Job drawing, mm, ordinate dimensions from the low corner. One solid piece. Give positions to 0.01 mm unless a question says otherwise; leave off trailing zeros. Loops run counter-clockwise (first coordinate to the right, second up) from the corner with the lowest first, then second, coordinate; pieces in that order, holes last. Notation, with made-up numbers: M 35.5,58 L 65.5,58 A31 ccw 65.5,94 Z; hole C 47.5,-2.5 d9. An arc over 180 degrees is marked long. Put each result on its own line as item: value.
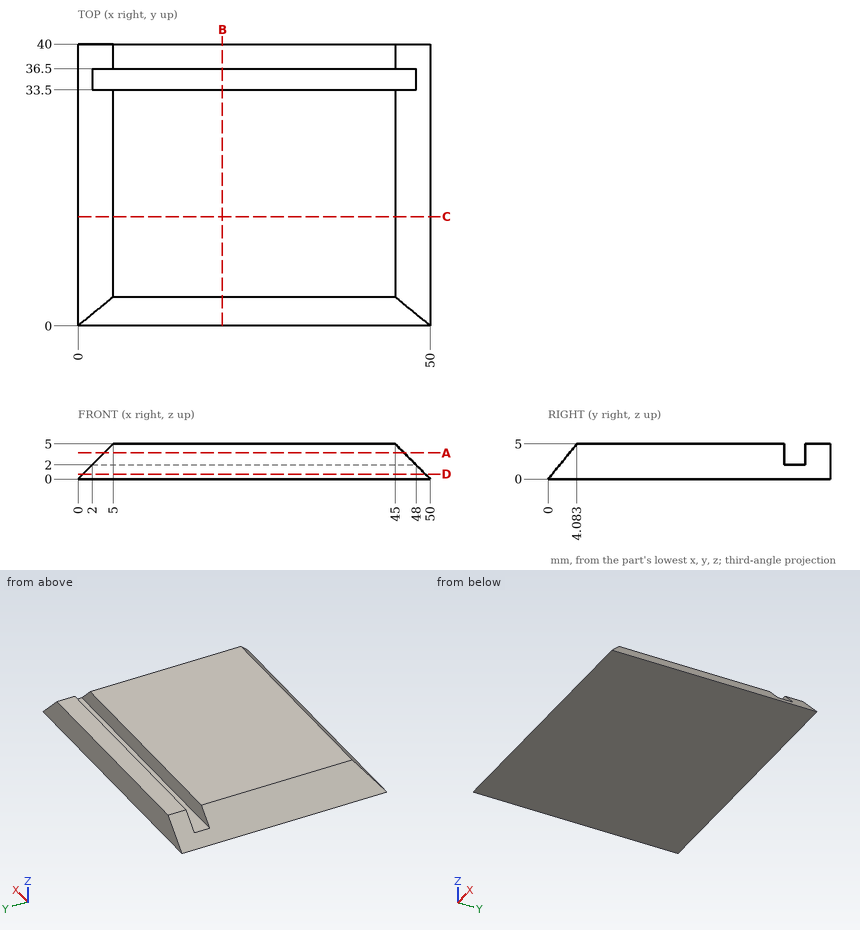
Q1. Slice it at A-A (z = 3.7). List the corners of the cut face in (x, y).
Here are the results:
outline: M 3.7,3.02 L 46.3,3.02 L 46.3,33.5 L 3.7,33.5 Z; M 3.7,36.5 L 46.3,36.5 L 46.3,40 L 3.7,40 Z
Q2. Slice it at D-D (z = 0.7). List the corners of the cut face in (x, y), and give its area (3 significant figures).
Here are the results:
outline: M 0.7,0.57 L 49.3,0.57 L 49.3,40 L 0.7,40 Z
area: 1,920 mm²
Q3. Probe line 1 (Z direction, x = 45, y = 34); line 2 (Y direction, x = 31.5, z = 2.25); line 3 (Y direction, x = 11.5, z = 3.9) (1 decimal). List the from-to ranges inside material, lowest first. Write a range as from..to.
Here are the results:
line 1: 0..2
line 2: 1.84..33.5, 36.5..40
line 3: 3.2..33.5, 36.5..40
Q4. Slice it at C-C (y = 15.5). List the corners of the cut face in (x, z).
Here are the results:
outline: M 0,0 L 50,0 L 45,5 L 5,5 Z
Q5. Slice it at B-B (x = 20.5). List the corners of the cut face in (y, z).
Here are the results:
outline: M 0,0 L 40,0 L 40,5 L 36.5,5 L 36.5,2 L 33.5,2 L 33.5,5 L 4.08,5 Z
Q6. Drop flat-ended pins along their axis: pin 1 Ø1.5 at (x, z) = (24.5, 2.5) entering from -Y; pin 2 Ø2 at (x, z) = (13.5, 2) entering from -Y; pin 3 Ø0.9 at (x, y) = (19, 35) entering from +Z. Give the stop position or say it passes through.
Here are the results:
pin 1: y = 1.43
pin 2: y = 0.82
pin 3: z = 2
